from build123d import *
from build123d.topology import SkipClean

# Parameters (mm, degrees)
SKETCH1_R               = 22.5
SKETCH1_R_2             = 9.525
BOSS_EXTRUDE1_DEPTH     = 95
SKETCH2_OUTSIDE_W       = 69.87
SKETCH2_OUTSIDE_H       = 69.87
SKETCH2_OUTSIDE_R       = 15
CUT_EXTRUDE1_DEPTH      = 50
SKETCH4_OUTSIDE_W       = 69.87
SKETCH4_OUTSIDE_H       = 69.87
SKETCH4_OUTSIDE_R       = 17.5
CUT_EXTRUDE2_DEPTH      = 37
SKETCH11_OUTSIDE_W      = 69.87
SKETCH11_OUTSIDE_H      = 69.87
SKETCH11_OUTSIDE_R      = 14.513
CUT_EXTRUDE3_DEPTH      = 5.88
SKETCH12_R              = 17.5
SKETCH12_R_2            = 9.525
BOSS_EXTRUDE2_DEPTH     = 203.2
BOSS_EXTRUDE3_START     = 15
SKETCH13_R              = 14.513
SKETCH13_R_2            = 9.525
BOSS_EXTRUDE3_DEPTH     = 15
SKETCH15_OUTSIDE_W      = 110.92
SKETCH15_OUTSIDE_H      = 110.92
SKETCH15_OUTSIDE_R      = 19.05
CUT_EXTRUDE5_DEPTH      = 251.231372933
SKETCH16_OUTSIDE_W      = 103.66
SKETCH16_OUTSIDE_H      = 103.66
SKETCH16_OUTSIDE_R      = 13.5
CUT_EXTRUDE6_DEPTH      = 2
FILLET2_R               = 0.396875
SKETCH17_R              = 17.5
CUT_EXTRUDE7_DEPTH      = 8.4
CUT_EXTRUDE8_DEPTH      = 292.049557636
CUT_EXTRUDE8_DEPTH_BACK = 292.049557636
SKETCH20_W              = 3.175
SKETCH20_H              = 25.4
FILLET3_R               = 3.175
CUT_EXTRUDE9_REACH      = 293.05
CUT_EXTRUDE9_END_RADIUS = 17.5
CUT_EXTRUDE10_REACH     = 307.988
SKETCH22_R              = 12.7


with BuildPart() as part:
    # Sketch1 → Boss-Extrude1 (new body)
    with BuildSketch(Plane(origin=(0, 0, 0), x_dir=(1, 0, 0), z_dir=(0, 1, 0))):
        with Locations(Location((0, 0, 0), (0, 0, 270))):
            Circle(SKETCH1_R)
        with Locations(Location((0, 0, 0), (0, 0, 270))):
            Circle(SKETCH1_R_2, mode=Mode.SUBTRACT)
    extrude(amount=BOSS_EXTRUDE1_DEPTH)

    # Sketch2 outside → Cut-Extrude1 (cut)
    with BuildSketch(Plane.XZ):
        Rectangle(SKETCH2_OUTSIDE_W, SKETCH2_OUTSIDE_H)
        with Locations(Location((0, 0, 0), (0, 0, 270))):
            Circle(SKETCH2_OUTSIDE_R, mode=Mode.SUBTRACT)
    extrude(amount=-CUT_EXTRUDE1_DEPTH, mode=Mode.SUBTRACT)

    # Sketch4 outside → Cut-Extrude2 (cut)
    with BuildSketch(Plane(origin=(0, 95, 0), x_dir=(1, 0, 0), z_dir=(0, 1, 0))):
        Rectangle(SKETCH4_OUTSIDE_W, SKETCH4_OUTSIDE_H)
        with Locations(Location((0, 0, 0), (0, 0, 270))):
            Circle(SKETCH4_OUTSIDE_R, mode=Mode.SUBTRACT)
    extrude(amount=-CUT_EXTRUDE2_DEPTH, mode=Mode.SUBTRACT)

    # Sketch11 outside → Cut-Extrude3 (cut)
    with BuildSketch(Plane.XZ):
        Rectangle(SKETCH11_OUTSIDE_W, SKETCH11_OUTSIDE_H)
        with Locations(Location((0, 0, 0), (0, 0, 270))):
            Circle(SKETCH11_OUTSIDE_R, mode=Mode.SUBTRACT)
    extrude(amount=-CUT_EXTRUDE3_DEPTH, mode=Mode.SUBTRACT)

    # Sketch12 → Boss-Extrude2 (add)
    with BuildSketch(Plane(origin=(0, 95, 0), x_dir=(1, 0, 0), z_dir=(0, 1, 0))):
        with Locations(Location((0, 0, 0), (0, 0, 270))):
            Circle(SKETCH12_R)
        with Locations(Location((0, 0, 0), (0, 0, 270))):
            Circle(SKETCH12_R_2, mode=Mode.SUBTRACT)
    extrude(amount=BOSS_EXTRUDE2_DEPTH)

    # Sketch13 → Boss-Extrude3 (add)
    with SkipClean():  # the faces are left unmerged after this step: merging them gives an invalid solid
        with BuildSketch(Plane.XZ.offset(BOSS_EXTRUDE3_START)):
            with Locations(Location((0, 0, 0), (0, 0, 270))):
                Circle(SKETCH13_R)
            with Locations(Location((0, 0, 0), (0, 0, 270))):
                Circle(SKETCH13_R_2, mode=Mode.SUBTRACT)
        extrude(amount=-BOSS_EXTRUDE3_DEPTH)

    # Sketch15 outside → Cut-Extrude5 (cut, through all)
    with SkipClean():  # the faces are left unmerged after this step: merging them gives an invalid solid
        with BuildSketch(Plane.XZ.offset(-50)):
            Rectangle(SKETCH15_OUTSIDE_W, SKETCH15_OUTSIDE_H)
            with Locations(Location((0, 0, 0), (0, 0, 270))):
                Circle(SKETCH15_OUTSIDE_R, mode=Mode.SUBTRACT)
        extrude(amount=-CUT_EXTRUDE5_DEPTH, mode=Mode.SUBTRACT)

    # Sketch16 outside → Cut-Extrude6 (cut)
    with SkipClean():  # the faces are left unmerged after this step: merging them gives an invalid solid
        with BuildSketch(Plane.XZ.offset(-5.88)):
            Rectangle(SKETCH16_OUTSIDE_W, SKETCH16_OUTSIDE_H)
            with Locations(Location((0, 0, 0), (0, 0, 270))):
                Circle(SKETCH16_OUTSIDE_R, mode=Mode.SUBTRACT)
        extrude(amount=CUT_EXTRUDE6_DEPTH, mode=Mode.SUBTRACT)

    # Fillet2
    fillet2_edges = [part.edges().sort_by_distance(p)[0] for p in [
        (0, 5.88, 13.5),
        (0, 3.88, 13.5),
    ]]
    fillet(fillet2_edges, radius=FILLET2_R)

    # Sketch17 → Cut-Extrude7 (cut)
    with BuildSketch(Plane(origin=(0, 298.2, 0), x_dir=(1, 0, 0), z_dir=(0, 1, 0))):
        with Locations(Location((0, 0, 0), (0, 0, 270))):
            Circle(SKETCH17_R)
    extrude(amount=-CUT_EXTRUDE7_DEPTH, mode=Mode.SUBTRACT)

    # Sketch20 → Cut-Extrude8 (cut, two sides: drawn at the far end of the back side and taken through both)
    with BuildSketch(Plane.XY.offset(-CUT_EXTRUDE8_DEPTH_BACK)):
        with Locations((-17.4625, 105.625)):
            Rectangle(SKETCH20_W, SKETCH20_H)
        with Locations((17.4625, 105.625)):
            Rectangle(SKETCH20_W, SKETCH20_H)
    extrude(amount=CUT_EXTRUDE8_DEPTH + CUT_EXTRUDE8_DEPTH_BACK, mode=Mode.SUBTRACT)

    # Fillet3
    # the kernel refuses this fillet: 3.175 mm, written as the material it adds along each edge
    with BuildSketch(Plane(origin=(-15.875, 92.925, 15.301899161), x_dir=(0, 1, 0), z_dir=(0, 0, -1))) as fillet3_piece_1_section:
        with BuildLine():
            CenterArc((FILLET3_R, -FILLET3_R), FILLET3_R, 90, 90)
            Line((0, -FILLET3_R), (0, 0))
            Line((0, 0), (FILLET3_R, 0))
        make_face()
    fillet3_piece_1 = extrude(amount=30.603798322, mode=Mode.PRIVATE)
    fillet3_piece_1 = fillet3_piece_1 & Plane(origin=(0, 93.819377515, 0), x_dir=(0, 0, 1), z_dir=(0, 1, 0)) * Cylinder(17.5, 74, mode=Mode.PRIVATE)
    add(fillet3_piece_1)
    with BuildSketch(Plane(origin=(-15.875, 118.325, 15.301899161), x_dir=(0, -1, 0), z_dir=(0, 0, -1))) as fillet3_piece_2_section:
        with BuildLine():
            CenterArc((FILLET3_R, FILLET3_R), FILLET3_R, 180, 90)
            Line((0, FILLET3_R), (0, 0))
            Line((0, 0), (FILLET3_R, 0))
        make_face()
    fillet3_piece_2 = extrude(amount=30.603798322, mode=Mode.PRIVATE)
    fillet3_piece_2 = fillet3_piece_2 & Plane(origin=(0, 117.430622485, 0), x_dir=(0, 0, 1), z_dir=(0, 1, 0)) * Cylinder(17.5, 74, mode=Mode.PRIVATE)
    add(fillet3_piece_2)
    with BuildSketch(Plane(origin=(15.875, 92.925, -15.301899161), x_dir=(0, 1, 0), z_dir=(0, 0, 1))) as fillet3_piece_3_section:
        with BuildLine():
            CenterArc((FILLET3_R, -FILLET3_R), FILLET3_R, 90, 90)
            Line((0, -FILLET3_R), (0, 0))
            Line((0, 0), (FILLET3_R, 0))
        make_face()
    fillet3_piece_3 = extrude(amount=30.603798322, mode=Mode.PRIVATE)
    fillet3_piece_3 = fillet3_piece_3 & Plane(origin=(0, 93.81935464, 0), x_dir=(0, 0, 1), z_dir=(0, 1, 0)) * Cylinder(17.5, 74, mode=Mode.PRIVATE)
    add(fillet3_piece_3)
    with BuildSketch(Plane(origin=(15.875, 118.325, -15.301899161), x_dir=(0, -1, 0), z_dir=(0, 0, 1))) as fillet3_piece_4_section:
        with BuildLine():
            CenterArc((FILLET3_R, FILLET3_R), FILLET3_R, 180, 90)
            Line((0, FILLET3_R), (0, 0))
            Line((0, 0), (FILLET3_R, 0))
        make_face()
    fillet3_piece_4 = extrude(amount=30.603798322, mode=Mode.PRIVATE)
    fillet3_piece_4 = fillet3_piece_4 & Plane(origin=(0, 117.43064536, 0), x_dir=(0, 0, 1), z_dir=(0, 1, 0)) * Cylinder(17.5, 74, mode=Mode.PRIVATE)
    add(fillet3_piece_4)

    # Cut-Extrude9: up to this cylinder (the profile starts inside it)
    cut_extrude9_end = Plane(origin=(0, 105.625, 0), z_dir=(0, 1, 0)) * Cylinder(CUT_EXTRUDE9_END_RADIUS, 622.1, mode=Mode.PRIVATE)
    # Sketch21 → Cut-Extrude9 (cut, up to the surface)
    with BuildSketch(Plane.XY, mode=Mode.PRIVATE) as cut_extrude9_sk1:
        with BuildLine():
            Line((-6.35, 99.275), (-6.35, 111.975))
            ThreePointArc((-6.35, 111.975), (0, 118.325), (6.35, 111.975))
            Line((6.35, 111.975), (6.35, 99.275))
            ThreePointArc((6.35, 99.275), (0, 92.925), (-6.35, 99.275))
        make_face()
    cut_extrude9_tool1 = extrude(cut_extrude9_sk1.sketch, amount=CUT_EXTRUDE9_REACH, mode=Mode.PRIVATE) & cut_extrude9_end
    add(cut_extrude9_tool1.solids().sort_by_distance((0, 105.625, 0))[0], mode=Mode.SUBTRACT)

    # Cut-Extrude10: up to this face of the body (flat: up to its plane)
    cut_extrude10_end = Plane(part.part.faces().sort_by_distance((0, -15, 14.102510371))[0])
    # Sketch22 → Cut-Extrude10 (cut, up to the picked face)
    with BuildSketch(Plane(origin=(0, 289.8, 0), x_dir=(1, 0, 0), z_dir=(0, 1, 0)), mode=Mode.PRIVATE) as cut_extrude10_sk1:
        with Locations(Location((0, 0, 0), (0, 0, 270))):
            Circle(SKETCH22_R)
    cut_extrude10_tool1 = split(extrude(cut_extrude10_sk1.sketch, amount=-CUT_EXTRUDE10_REACH, mode=Mode.PRIVATE), bisect_by=cut_extrude10_end, keep=Keep.BOTH, mode=Mode.PRIVATE)
    add(cut_extrude10_tool1.solids().sort_by(Axis((0, 289.8, 0), (0, -1, 0)))[0], mode=Mode.SUBTRACT)


solid = part.part
Source: CAD feature listing. Evaluate the final solid. Frame: model axes, mm. A direction names the side the tool comes from. Round coordinates to 2 decimals unless told otherwise and drop trailing zeros. Write each loop counter-clockwise with the first axis right and the second up, starting at its lowest first coordinate (ties: lowest second). Pieces come first, ordered by that corner, then holes. Notation, with made-up numbers: (46.5, 57.5) - (53.5, 57.5) arc R26 ccw to (53.5, 75.5) - close; hole circle Ø8 at (64.5, -24). An arc over 180 degrees is marked (long way). Use CSV: the item, a comma, the result in double quotes. Start each with the question number.
(1) Cut plane B-B, the plane y = 144. Return loops of the section in (x, z).
(2) Mould query, pull axis Y, two halves, no side actions, for faces 5 (the face through (-15.875, 105, 0)), 6 (the face through (-11.59, 53.94, 15.12)), 7 (the face through (-13, -15, 0)). Classes: pulls with the +Y half, pulls with the -Y half, needs draft (parallel to the pull), parting line crosses it, or undercut.
(3) Set-up query: faces 1 (the face through (-13.18, 4.89, 2.93)), 2 (the face through (15.875, 105, 0)), 3 (the face through (0.66, 27.631, 14.985)), 4 (the face through (-0.14, 118.323, 14.204)). Return all of +Z, -Z, +X, -X, +Y, -Y with unobstructed straight access to the full face (end or side cutting, diameter ignored); none if empty.
(4) First-contact query: pin 1 Ø1.6 at (y, z) = (104, 12.5) entering from +X; pin 2 Ø8.5 at (x, z) = (-6, 0) entering from +Y; pin 3 Ø11.5 at (x, z) = (8.5, -4.5) entering from +Y; pin 4 Ø10 at (x, y) = (14, 160.5) entering from -Z. Flat tips, straight axial feed; report the tip coordinate or a pass-through.
(5) Material intervals for probe 1 along X at (y, z) = (84.5, 0); probe 2 along Y at (x, z) = (11.5, 8); probe 3 along Y at (x, z) = (9.5, 16), sorted ascending. Write a range as [from, to].
(6) Cut plane A-A, the plane x = 0. Give the number of separate pieces and of enclosed holes in the cut face, and give its area (3 significant figures).
Geometry says:
1,outline,"circle Ø35 at (0, 0); hole circle Ø25.4 at (0, 0)"
2,face 5,"undercut"
2,face 6,"needs draft"
2,face 7,"pulls with the -Y half"
3,face 1,"none"
3,face 2,"+Z, -Z, +X"
3,face 3,"-Y"
3,face 4,"+Z"
4,pin 1,"x = 13.01"
4,pin 2,"through"
4,pin 3,"y = 289.8"
4,pin 4,"z = -15.01"
5,probe 1,"[-17.5, -12.7], [12.7, 17.5]"
5,probe 2,"[-15, 3.88], [5.88, 289.8]"
5,probe 3,"[50, 58]"
6,separate pieces,"3"
6,enclosed holes,"0"
6,area,"2,480 mm²"
